```python
from build123d import *

# Parameters (mm, degrees)
BOSS_EXTRUDE1_DEPTH    = 20
SKETCH2_R              = 10
CUT_EXTRUDE1_DEPTH     = 20
SPUR_START             = 143.992112376
SPUR_GEAR_AM_OUTLINE_R = 5
SPUR_GEAR_AM_DEPTH     = 10
SKETCH4_R              = 40
BOSS_EXTRUDE2_DEPTH    = 20
BOSS_EXTRUDE3_DEPTH    = 20
SKETCH5_R              = 20
CUT_EXTRUDE4_DEPTH     = 20
BOSS_EXTRUDE4_START    = -40
SKETCH8_R              = 10
BOSS_EXTRUDE4_DEPTH    = 40


# Read off the part's stored shape, not the designer's step: spur gear_am
with BuildPart() as part:
    # Sketch1 → Boss-Extrude1 (new body)
    with BuildSketch(Plane.XY):
        with BuildLine():
            Line((-220, 20), (220, 20))
            ThreePointArc((220, 20), (240, 0), (220, -20))
            Line((220, -20), (-220, -20))
            ThreePointArc((-220, -20), (-240, 0), (-220, 20))
        make_face()
    extrude(amount=BOSS_EXTRUDE1_DEPTH)

    # Sketch2 → Cut-Extrude1 (cut)
    with BuildSketch(Plane.XY.offset(20)):
        with Locations((220, 0)):
            Circle(SKETCH2_R)
        with Locations((-220, 0)):
            Circle(SKETCH2_R)
    extrude(amount=-CUT_EXTRUDE1_DEPTH, mode=Mode.SUBTRACT)

    # Sketch4 → Boss-Extrude2 (add)
    with BuildSketch(Plane.XY.offset(20)):
        with Locations((220, 0)):
            Circle(SKETCH4_R)
    extrude(amount=-BOSS_EXTRUDE2_DEPTH)

    # Sketch6 → Boss-Extrude3 (add)
    with BuildSketch(Plane.XY.offset(20)):
        Polygon((-220, -20), (-220, -30.112160349), (-209.887839651, -20), align=None)
        Polygon((-209.887839651, 20), (-220, 20), (-220, 30.112160349), align=None)
    extrude(amount=-BOSS_EXTRUDE3_DEPTH)

    # Sketch5 → Cut-Extrude4 (cut)
    with BuildSketch(Plane(origin=(0, 0, 0), x_dir=(-1, 0, 0), z_dir=(0, 0, -1))):
        with Locations((-220, 0)):
            Circle(SKETCH5_R)
    extrude(amount=-CUT_EXTRUDE4_DEPTH, mode=Mode.SUBTRACT)

    # Sketch8 → Boss-Extrude4 (add)
    with BuildSketch(Plane(origin=(0, 0, 0), x_dir=(-1, 0, 0), z_dir=(0, 0, -1)).offset(BOSS_EXTRUDE4_START)):
        with Locations((220, 0)):
            Circle(SKETCH8_R)
    extrude(amount=BOSS_EXTRUDE4_DEPTH)


with BuildPart() as body_2:
    # spur gear_am outline → spur gear_am (new body)
    with BuildSketch(Plane.YZ.offset(SPUR_START)):
        with BuildLine():
            ThreePointArc((13.133221577, -371.123184299), (13.390101578, -371.125934087), (13.646981578, -371.123184299))
            ThreePointArc((13.646981578, -371.123184299), (14.846401327, -368.975865304), (14.562642986, -366.532697728))
            ThreePointArc((14.562642986, -366.532697728), (15.707420018, -366.257906902), (16.795082087, -365.807334294))
            ThreePointArc((16.795082087, -365.807334294), (18.001574637, -367.950687351), (20.234088035, -368.982903671))
            ThreePointArc((20.234088035, -368.982903671), (20.443524605, -368.834138019), (20.649728607, -368.680923118))
            ThreePointArc((20.649728607, -368.680923118), (20.35791713, -366.238704319), (18.69229394, -364.428929198))
            ThreePointArc((18.69229394, -364.428929198), (19.456920018, -363.533735693), (20.072017182, -362.529903073))
            ThreePointArc((20.072017182, -362.529903073), (22.307921476, -363.554753593), (24.720784284, -363.077595687))
            ThreePointArc((24.720784284, -363.077595687), (24.802779773, -362.834138019), (24.879544856, -362.588980889))
            ThreePointArc((24.879544856, -362.588980889), (23.207964219, -360.78470686), (20.796687626, -360.299596778))
            ThreePointArc((20.796687626, -360.299596778), (20.889101578, -359.125934087), (20.796687626, -357.952271396))
            ThreePointArc((20.796687626, -357.952271396), (23.207964219, -357.467161313), (24.879544856, -355.662887284))
            ThreePointArc((24.879544856, -355.662887284), (24.802779773, -355.417730154), (24.720784284, -355.174272487))
            ThreePointArc((24.720784284, -355.174272487), (22.307921476, -354.697114581), (20.072017182, -355.7219651))
            ThreePointArc((20.072017182, -355.7219651), (19.456920018, -354.71813248), (18.69229394, -353.822938975))
            ThreePointArc((18.69229394, -353.822938975), (20.35791713, -352.013163854), (20.649728607, -349.570945055))
            ThreePointArc((20.649728607, -349.570945055), (20.443524605, -349.417730154), (20.234088035, -349.268964503))
            ThreePointArc((20.234088035, -349.268964503), (18.001574638, -350.301180822), (16.795082087, -352.444533879))
            ThreePointArc((16.795082087, -352.444533879), (15.707420018, -351.993961271), (14.562642986, -351.719170445))
            ThreePointArc((14.562642986, -351.719170445), (14.846401327, -349.276002869), (13.646981578, -347.128683874))
            ThreePointArc((13.646981578, -347.128683874), (13.390101577, -347.125934087), (13.133221577, -347.128683874))
            ThreePointArc((13.133221577, -347.128683874), (11.933801828, -349.276002869), (12.217560169, -351.719170445))
            ThreePointArc((12.217560169, -351.719170445), (11.072783137, -351.993961271), (9.985121068, -352.444533879))
            ThreePointArc((9.985121068, -352.444533879), (8.778628518, -350.301180823), (6.546115121, -349.268964503))
            ThreePointArc((6.546115121, -349.268964503), (6.33667855, -349.417730154), (6.130474548, -349.570945055))
            ThreePointArc((6.130474548, -349.570945055), (6.422286026, -352.013163854), (8.087909215, -353.822938975))
            ThreePointArc((8.087909215, -353.822938975), (7.323283137, -354.71813248), (6.708185973, -355.7219651))
            ThreePointArc((6.708185973, -355.7219651), (4.472281679, -354.697114581), (2.059418871, -355.174272487))
            ThreePointArc((2.059418871, -355.174272487), (1.977423382, -355.417730154), (1.900658299, -355.662887284))
            ThreePointArc((1.900658299, -355.662887284), (3.572238937, -357.467161313), (5.98351553, -357.952271396))
            ThreePointArc((5.98351553, -357.952271396), (5.891101578, -359.125934087), (5.98351553, -360.299596778))
            ThreePointArc((5.98351553, -360.299596778), (3.572238937, -360.78470686), (1.900658299, -362.588980889))
            ThreePointArc((1.900658299, -362.588980889), (1.977423382, -362.834138019), (2.059418871, -363.077595687))
            ThreePointArc((2.059418871, -363.077595687), (4.472281679, -363.554753593), (6.708185973, -362.529903073))
            ThreePointArc((6.708185973, -362.529903073), (7.323283137, -363.533735693), (8.087909215, -364.428929198))
            ThreePointArc((8.087909215, -364.428929198), (6.422286026, -366.23870432), (6.130474548, -368.680923118))
            ThreePointArc((6.130474548, -368.680923118), (6.33667855, -368.834138019), (6.546115121, -368.982903671))
            ThreePointArc((6.546115121, -368.982903671), (8.778628518, -367.950687351), (9.985121068, -365.807334294))
            ThreePointArc((9.985121068, -365.807334294), (11.072783137, -366.257906902), (12.217560169, -366.532697728))
            ThreePointArc((12.217560169, -366.532697728), (11.933801828, -368.975865304), (13.133221577, -371.123184299))
        make_face()
        with Locations((13.390101578, -359.125934087)):
            Circle(SPUR_GEAR_AM_OUTLINE_R, mode=Mode.SUBTRACT)
    extrude(amount=SPUR_GEAR_AM_DEPTH)


solid = part.part
```
CAD build for the part. Positions are in the model's coordinates, mm. A direction names the side the tool comes from. Coordinates: 2 decimals unless noted, no trailing zeros. Write each loop counter-clockwise with the first axis right and the second up, starting at its lowest first coordinate (ties: lowest second). Pieces come first, ordered by that corner, then holes. Notation, with made-up numbers: (-36, 21) -> (-29, 21) arc R12 cw to (-29, 40) -> close; hole circle Ø10 at (60, 60). An arc over 180 degrees is marked (long way). Return JSON: item names as keys, results as strings. Group by question number.
Q1. Flat gauge pins, fed straight in: pin 1 (5 mm diameter, centred on y = 26.5, z = 14, fed in from -X); pin 2 (16 mm diameter, centred on x = -80, z = 8, fed in from -Y); pin 3 (10 mm diameter, centred on x = 130, y = -15, fed in from +Z). Where does each tip first touch, or does it go through?
Q2. Cut at C-C, the plane z = 26.5. Give the cut face in (x, y).
Q3. Cut at D-D, the plane x = -90. Give the cut face in (y, z), then the cut area to 3 significant figures.
Q4. Cut at B-B, the plane x = 220. Give the cut face in (y, z).
Q5. Drill centre lines: line 1 (Y direction, x = 220, z = 7.75); line 2 (X direction, y = -3.5, z = 14.5); line 3 (Y direction, x = -186.5, z = 19.5). Where is each one in solid material? Low to high.
Q6. Cut at A-A, the plane y = 0. Give the cut face in (x, z), then the cut area to 3 significant figures.
Q7. Which spindle directions (+Z, -Z, +X, -X, +Y, -Y) get a long thin tool onto all of the face, cutting with end or side? Do faces 4 (the face through (-15, 20, 10)), 5 (the face through (-9, -20, 10)), 6 (the face through (-220, 25, 10)), 7 (the face through (-220, 0, 40)), 8 (the face through (7, 1, 0)). Say none if no direction does.
Q8. Pull direction X, two halves, no side cores. Call faces 1 (the face through (-215.015, 25.127, 10.14)), 2 (the face through (-229.237, -3.83, 30.14)), 3 (the face through (-220, -25, 10)): released by +X, released by -X, zero draft, split by the parting line, or undercut.
Returned:
{
 "1": {"pin 1": "stops at x = -220", "pin 2": "stops at y = -20", "pin 3": "stops at z = 20"},
 "2": {"outline": "circle Ø20 at (-220, 0)"},
 "3": {"outline": "(-20, 0) -> (20, 0) -> (20, 20) -> (-20, 20) -> close", "area": "800 mm2"},
 "4": {"outline": "(-40, 0) -> (-20, 0) -> (-20, 20) -> (-40, 20) -> close; (20, 0) -> (40, 0) -> (40, 20) -> (20, 20) -> close"},
 "5": {"line 1": "y = -40 to -20, 20 to 40", "line 2": "x = -239.69 to 200.31, 239.69 to 259.85", "line 3": "y = -20 to 20"},
 "6": {"outline": "(-240, 0) -> (200, 0) -> (200, 20) -> (-210, 20) -> (-210, 40) -> (-230, 40) -> (-230, 20) -> (-240, 20) -> close; (240, 0) -> (260, 0) -> (260, 20) -> (240, 20) -> close", "area": "9,600 mm2"},
 "7": {"face 4": "+Z, -Z, +Y", "face 5": "+Z, -Z, -Y", "face 6": "+Z, -Z, -X, +Y", "face 7": "+Z, +X, -X, +Y, -Y", "face 8": "-Z, +X, -X, +Y, -Y"},
 "8": {"face 1": "undercut", "face 2": "split by the parting line", "face 3": "released by -X"}
}
